The model under review builds one solid part; all positions refer to its coordinate system, in mm. A direction names the side the tool comes from. Coordinates: 2 decimals unless noted, no trailing zeros. Order: outer loops, then holes, each group sorted by start corner. A loop starts at its lowest first (then second) coordinate and runs counter-clockwise, first axis right, second up.
from build123d import *

# Parameters (mm, degrees)
SWEEP5_PROFILE_R         = 12.7
SKETCH70_W               = 38.1
SKETCH70_H               = 50.8
BOSS_EXTRUDE1_DEPTH      = 5
SKETCH71_W               = 38.1
SKETCH71_H               = 6
BOSS_EXTRUDE2_DEPTH      = 76.2
SKETCH72_W               = 6
SKETCH72_H               = 38.1
BOSS_EXTRUDE3_DEPTH      = 76.2
BOSS_EXTRUDE4_DEPTH      = 12.7
BOSS_EXTRUDE4_DEPTH_BACK = 50.8
SKETCH73_R               = 9.509112568
SKETCH74_R               = 12.5
BOSS_EXTRUDE5_DEPTH      = 5
FILLET1_R                = 2


with BuildPart() as part:
    # Sweep5: sweep along a path in Sketch47
    with BuildLine(Plane.XY) as sweep5_path:
        ThreePointArc((-9.644129197, -154.699679289), (106.137081113, -112.95981592), (155, 0))
    # Sweep5 profile (on start of the path) → Sweep5 (sweep)
    with BuildSketch(Plane(origin=(-9.644129197, -154.699679289, 0), x_dir=(0.06222018836928112, 0.9980624470238779, 0), z_dir=(0.9980624470238779, -0.06222018836928112, 0))):
        Circle(SWEEP5_PROFILE_R)
    sweep(path=sweep5_path.line)

    # Sketch70 → Boss-Extrude1 (add)
    with BuildSketch(Plane(origin=(0, 0, 0), x_dir=(0, 0, 1), z_dir=(-0.9980624470238779, 0.0622201883692814, 0))):
        with Locations((0, -153.127799021)):
            Rectangle(SKETCH70_W, SKETCH70_H)
    extrude(amount=BOSS_EXTRUDE1_DEPTH)

    # Sketch71 → Boss-Extrude2 (add)
    with BuildSketch(Plane(origin=(-4.990312235, 0.311100942, 0), x_dir=(0, 0, 1), z_dir=(-0.9980624470238779, 0.0622201883692814, 0))):
        with Locations((0, -175.527799021)):
            Rectangle(SKETCH71_W, SKETCH71_H)
    extrude(amount=BOSS_EXTRUDE2_DEPTH)

    # Sketch72 → Boss-Extrude3 (add)
    with BuildSketch(Plane(origin=(-10.734712154, -172.19351727, 0), x_dir=(0.9980624470238779, -0.0622201883692814, 0), z_dir=(0.0622201883692814, 0.9980624470238779, 0))):
        with Locations((-78.2, 0)):
            Rectangle(SKETCH72_W, SKETCH72_H)
    extrude(amount=BOSS_EXTRUDE3_DEPTH)

    # Sketch73 → Boss-Extrude4 (add, two sides: drawn at the far end of the back side and taken through both)
    with BuildSketch(Plane(origin=(-81.042670698, 5.052279296, 0), x_dir=(0, 0, 1), z_dir=(-0.9980624470238779, 0.06222018836928128, 0)).offset(-BOSS_EXTRUDE4_DEPTH_BACK)):
        with Locations(Location((0, -144.487448774, 0), (0, 0, 270))):
            Circle(SKETCH73_R)
    extrude(amount=BOSS_EXTRUDE4_DEPTH + BOSS_EXTRUDE4_DEPTH_BACK)

    # Sketch74 → Boss-Extrude5 (add)
    with BuildSketch(Plane(origin=(-93.718063776, 5.842475688, 0), x_dir=(0, 0, 1), z_dir=(-0.9980624470238779, 0.06222018836928128, 0))):
        with Locations(Location((0, -144.487448774, 0), (0, 0, 270))):
            Circle(SKETCH74_R)
    extrude(amount=BOSS_EXTRUDE5_DEPTH)

    # Fillet1
    fillet1_edges = [part.edges().sort_by_distance(p)[0] for p in [
        (-106.920659936, -125.578139471, 0),
    ]]
    fillet(fillet1_edges, radius=FILLET1_R)


solid = part.part
(1) Wall thickness on line 1 (Z direction, x = 147, y = -50.5); line 2 (Y direction, x = -52, z = 4); line 3 (Y direction, x = -53, z = 0): over which ranges is each line inside the solid? List them lowest first.
(2) The part is to be moulded in two halves that separate along Y. For faces 1 (the face through (-89.63, -132.68, -8.2)), 2 (the face through (-84.084, -91.273, -0.267)), 3 (the face through (-104.926, -150.173, 3.755)), say which applies: +Y half, -Y half, draft (parallel to the pull), parting line (faces both ways), or undercut.
(3) Consider section A-A (z = -15.5). Give the boundary of the cut face in (x, y).
(4) Tool access review of faces 4 (the face through (-102.877, -141.079, 9.318)), 5 (the face through (-55, -171, -19.05)), 6 (the face through (-14.31, -149.21, -0.27)), 7 (the face through (-50.27, -169.73, -0.27)): name each direction out of +Z, -Z, +X, -X, +Y, -Y from which nothing blocks a thin tool from reaching the whole face with its end or side.
(5) Insertion check: pin 1 Ø1.5 at (x, y) = (38, -150.5) entering from -Z; pin 2 Ø1 at (y, z) = (-38.5, -9) entering from +X; pin 3 Ø12 at (y, z) = (-118.5, -5.5) entering from -X. Each pin has a flat end and moves straight along its axis. Give the tip position at first contact, or say it passes through.
Findings:
1. line 1: z = -12.69 to 12.69
1. line 2: y = -175.63 to -169.62, -150.17 to -132.88
1. line 3: y = -175.57 to -169.56, -150.99 to -131.94
2. face 1: undercut
2. face 2: +Y half
2. face 3: parting line
3. outline: (-92.15, -173.13) - (-11.11, -178.18) - (-7.95, -127.48) - (-12.94, -127.17) - (-15.73, -171.88) - (-85.79, -167.51) - (-81.05, -91.46) - (-87.04, -91.09) - close
4. face 4: none
4. face 5: -Z, +X, -X, +Y, -Y
4. face 6: +Z, -Z, +Y
4. face 7: +Z, -Z
5. pin 1: stops at z = -12.7
5. pin 2: stops at x = 159.88
5. pin 3: stops at x = -89.12
